```python
from build123d import *


with BuildPart() as part:
    # Sketch1 → Revolve1 (revolve)
    with BuildSketch(Plane.XY):
        with BuildLine():
            Line((0, 0), (7.62, 0))
            Line((7.62, 0), (7.62, 6.726876964))
            Line((7.62, 6.726876964), (10.903948776, 3.442928188))
            ThreePointArc((10.903948776, 3.442928188), (12.7, 2.698979412), (14.496051224, 3.442928188))
            Line((14.496051224, 3.442928188), (17.78, 6.726876964))
            Line((17.78, 6.726876964), (17.78, 0))
            Line((17.78, 0), (25.4, 0))
            Line((25.4, 0), (25.4, -3.9624))
            Line((25.4, -3.9624), (0, -3.9624))
            Line((0, -3.9624), (0, 0))
        make_face()
    revolve(axis=Axis((25.4, -3.9624, 0), (-1, 0, 0)))


solid = part.part
```
Geometry: final body of the model. Coordinates: model frame, mm. A direction names the side the tool comes from. Round coordinates to 2 decimals unless told otherwise and drop trailing zeros. Write each loop counter-clockwise with the first axis right and the second up, starting at its lowest first coordinate (ties: lowest second). Pieces come first, ordered by that corner, then holes. Notation, with made-up numbers: (-13, -0.75) -> (-6, -0.75) arc R21 cw to (-6, 14.25) -> close; hole circle Ø11 at (17, 13). An arc over 180 degrees is marked (long way). Use CSV: the item, a comma, the result in double quotes. Start each with the question number.
Q1. Pull-direction query (X, two-part tool) for faces 4 (the face through (17.78, 1, 0)), 5 (the face through (21.643, -0.183, -1.19)), 6 (the face through (0, -4, 0)), 7 (the face through (14.701, 3.297, -2.286)); classes: pulls with the +X half, pulls with the -X half, needs draft (parallel to the pull), parting line crosses it, or undercut.
Q2. Section A-A (z = 0). Return loops of the section in (x, y), plus the area to 3 significant figures.
Q3. Reachability of faces 1 (the face through (25.4, -4, 0)), 2 (the face through (10.744, -5.602, 7.385)), 3 (the face through (7.62, -9, 0)) from +Z, -Z, +X, -X, +Y, -Y: full face, straight path, thin tool, end or side. Return the list, or none.
Q4. Section B-B (x = 20). Return loops of the section in (y, z), plus the area to 3 significant figures.
Q5. Section C-C (x = 13.5). Return loops of the section in (y, z).
Q6. First-contact query: pin 1 Ø1 at (x, z) = (5.5, 1.5) entering from +Y; pin 2 Ø3 at (x, z) = (20.5, -5.5) entering from +Y; pin 3 Ø2 at (y, z) = (-4.5, -8) entering from -X; pin 4 Ø8 at (y, z) = (-7.5, -8) entering from +X. Flat tips, straight axial feed; report the tip coordinate or a pass-through.
Q7. Line query: L1, parallel to Z at x = 22.75, y = -4; L2, parallel to X at y = -10.5, z = -7; L3, parallel to X at y = -12, z = 3.5. Output: solid intervals per line, ascending.
Result sheet:
1,face 4,"pulls with the +X half"
1,face 5,"needs draft"
1,face 6,"pulls with the -X half"
1,face 7,"undercut"
2,outline,"(0, -7.92) -> (7.62, -7.92) -> (7.62, -14.65) -> (10.9, -11.37) arc R2.54 cw to (14.5, -11.37) -> (17.78, -14.65) -> (17.78, -7.92) -> (25.4, -7.92) -> (25.4, 0) -> (17.78, 0) -> (17.78, 6.73) -> (14.5, 3.44) arc R2.54 cw to (10.9, 3.44) -> (7.62, 6.73) -> (7.62, 0) -> (0, 0) -> close"
2,area,"289 mm²"
3,face 1,"+Z, -Z, +X, +Y, -Y"
3,face 2,"none"
3,face 3,"-X"
4,outline,"circle Ø7.92 at (-3.96, 0)"
4,area,"49.3 mm²"
5,outline,"circle Ø13.58 at (-3.96, 0)"
6,pin 1,"y = -0.13"
6,pin 2,"through"
6,pin 3,"x = 7.62"
6,pin 4,"x = 17.78"
7,L1,"-3.96 to 3.96"
7,L2,"7.62 to 8.73, 16.67 to 17.78"
7,L3,"7.62 to 9.54, 15.86 to 17.78"
